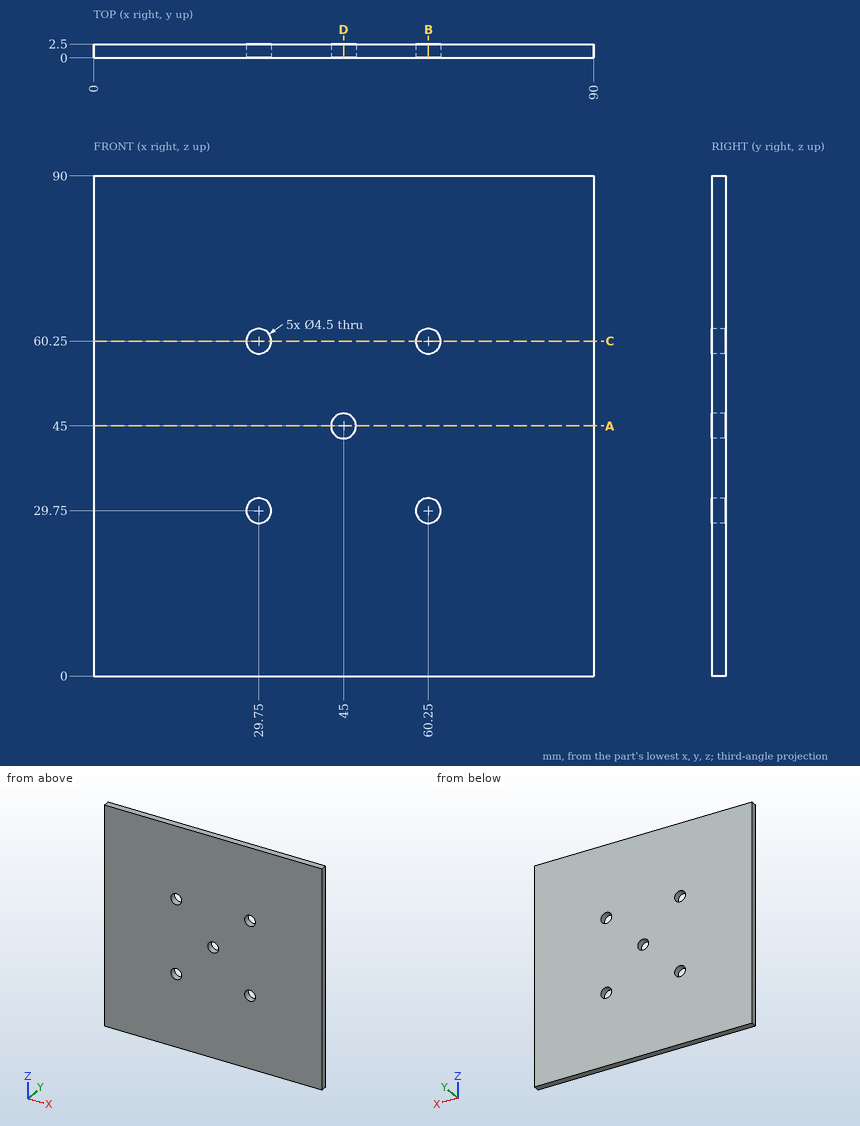
Input: dimensioned drawing with shaded views. Units: mm. Origin: part minimum x, y, z. Coordinates: 2 decimals unless noted, no trailing zeros. Order: outer loops, then holes, each group sorted by start corner. A loop starts at its lowest first (then second) coordinate and runs counter-clockwise, first axis right, second up. Notation, with made-up numbers: (-2, 11) - (10, 11) arc R19 cw to (10, 27) - close; hole circle Ø4 at (29, 65.25). An arc over 180 degrees is marked (long way). Put each result on its own line as item: value.
1. Cut plane A-A on z = 45. Return the cut outline in (x, y), then the cut area to 3 significant figures.
Report:
outline: (0, 0) - (42.75, 0) - (42.75, 2.5) - (0, 2.5) - close; (47.25, 0) - (90, 0) - (90, 2.5) - (47.25, 2.5) - close
area: 214 mm2
2. Line query: line 1 along X through (y, z) = (1.4, 29.75); line 2 along X through (y, z) = (1.4, 45). Output: solid intervals per line, ascending.
Report:
line 1: x = 0 to 27.5, 32 to 58, 62.5 to 90
line 2: x = 0 to 42.75, 47.25 to 90
3. Cut plane C-C on z = 60.25. Return the cut outline in (x, y).
Report:
outline: (0, 0) - (27.5, 0) - (27.5, 2.5) - (0, 2.5) - close; (32, 0) - (58, 0) - (58, 2.5) - (32, 2.5) - close; (62.5, 0) - (90, 0) - (90, 2.5) - (62.5, 2.5) - close
4. Cut plane B-B on x = 60.25. Return the cut outline in (y, z), then the cut area to 4 significant figures.
Report:
outline: (0, 0) - (2.5, 0) - (2.5, 27.5) - (0, 27.5) - close; (0, 32) - (2.5, 32) - (2.5, 58) - (0, 58) - close; (0, 62.5) - (2.5, 62.5) - (2.5, 90) - (0, 90) - close
area: 202.5 mm2
5. Cut plane D-D on x = 45. Return the cut outline in (y, z), then the cut area to 3 significant figures.
Report:
outline: (0, 0) - (2.5, 0) - (2.5, 42.75) - (0, 42.75) - close; (0, 47.25) - (2.5, 47.25) - (2.5, 90) - (0, 90) - close
area: 214 mm2
6. Contact query for a flat-ended pin moving along its axis: pin 1 Ø3.5 at (x, z) = (29.75, 29.75) entering from +Y. Output: stop coordinate, or through.
Report:
pin 1: passes through
